Verification items for this drawing (mm, ordinates from the low corner). Round coordinates to 2 decimals unless told otherwise and drop trailing zeros. Write each loop counter-clockwise with the first axis right and the second up, starting at its lowest first coordinate (ties: lowest second). Pieces come first, ordered by that corner, then holes.
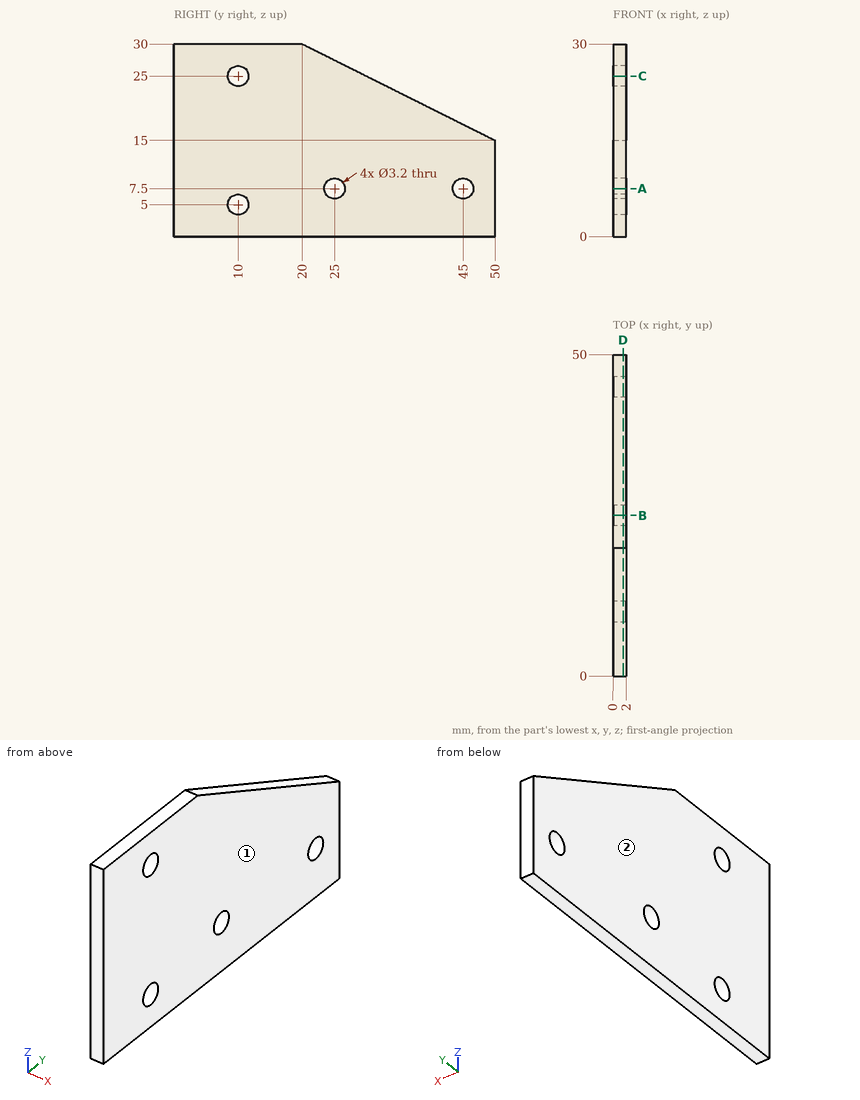
1. Section check D-D (x = 1.55). Record the cut outline in (y, z), plus the area to 3 significant figures.
2. Section check C-C (z = 25). Record the cut outline in (x, y).
3. Section check A-A (z = 7.5). Record the cut outline in (x, y), plus the area to 3 significant figures.
4. Scan lines: line 1 along Y through (x, z) = (1.05, 7.5); line 2 along Z through (x, y) = (1.35, 10); line 3 along Y through (x, z) = (1.15, 25). Record each from-to range of solid material in increasing order.
5. Depth check by flat-ended pin: pin 1 Ø1 at (x, y) = (1.5, 44) entering from +Z; pin 2 Ø3.5 at (y, z) = (45, 7.5) entering from -X; pin 3 Ø1.9 at (y, z) = (10, 5) entering from -X. Enter the tip coordinate at first touch or a pass-through.
6. Section check B-B (y = 25). Record the cut outline in (x, z), plus the area to 3 significant figures.
7. Release check for a two-part mould opening along X. For the marked faces 1 and 2 record: +X half, -X half, draft (parallel to the pull), parting line (faces both ways), or undercut.
Results below:
1. outline: (0, 0) - (50, 0) - (50, 15) - (20, 30) - (0, 30) - close; hole circle Ø3.2 at (10, 5); hole circle Ø3.2 at (10, 25); hole circle Ø3.2 at (25, 7.5); hole circle Ø3.2 at (45, 7.5)
1. area: 1,240 mm2
2. outline: (0, 0) - (2, 0) - (2, 8.4) - (0, 8.4) - close; (0, 11.6) - (2, 11.6) - (2, 30) - (0, 30) - close
3. outline: (0, 0) - (2, 0) - (2, 23.4) - (0, 23.4) - close; (0, 26.6) - (2, 26.6) - (2, 43.4) - (0, 43.4) - close; (0, 46.6) - (2, 46.6) - (2, 50) - (0, 50) - close
3. area: 87.2 mm2
4. line 1: y = 0 to 23.4, 26.6 to 43.4, 46.6 to 50
4. line 2: z = 0 to 3.4, 6.6 to 23.4, 26.6 to 30
4. line 3: y = 0 to 8.4, 11.6 to 30
5. pin 1: stops at z = 18.25
5. pin 2: stops at x = 0
5. pin 3: passes through
6. outline: (0, 0) - (2, 0) - (2, 5.9) - (0, 5.9) - close; (0, 9.1) - (2, 9.1) - (2, 27.5) - (0, 27.5) - close
6. area: 48.6 mm2
7. face 1: +X half
7. face 2: -X half
